Source: CAD feature listing. Evaluate the final solid. Frame: model axes, mm. Give positions to 0.01 mm unless a question says otherwise; leave off trailing zeros. Order: outer loops, then holes, each group sorted by start corner. A loop starts at its lowest first (then second) coordinate and runs counter-clockwise, first axis right, second up.
from build123d import *

# Parameters (mm, degrees)
BOSS_EXTRUDE1_DEPTH      = 5
SKETCH2_W                = 5
SKETCH2_H                = 22.5
BOSS_EXTRUDE2_DEPTH      = 38
SKETCH5_W                = 25
SKETCH5_H                = 5
BOSS_EXTRUDE3_DEPTH      = 30
FILLET3_R                = 5
SKETCH6_R                = 3
CUT_EXTRUDE4_DEPTH       = 172
SKETCH7_W                = 5
SKETCH7_H                = 22.5
BOSS_EXTRUDE4_DEPTH      = 51.5
SKETCH3_R                = 1.3
CUT_EXTRUDE2_DEPTH       = 357.71872673
SKETCH9_W                = 116
SKETCH9_H                = 63.779574991
CUT_EXTRUDE6_DEPTH       = 10
SKETCH10_W               = 25
SKETCH10_H               = 5
BOSS_EXTRUDE5_DEPTH      = 70
BOSS_EXTRUDE6_DEPTH      = 25
SKETCH12_W               = 25
SKETCH12_H               = 5
BOSS_EXTRUDE7_DEPTH      = 19.72
BOSS_EXTRUDE8_DEPTH      = 15
BOSS_EXTRUDE8_DEPTH_BACK = 4
CUT_EXTRUDE7_DEPTH       = 15
SKETCH15_R               = 2.25
CUT_EXTRUDE8_DEPTH       = 20
SKETCH16_W               = 6
SKETCH16_H               = 3
BOSS_EXTRUDE9_DEPTH      = 12.4
SKETCH17_R               = 1
CUT_EXTRUDE9_DEPTH       = 282.347152812
SKETCH27_W               = 25.232191294
SKETCH27_H               = 19
BOSS_EXTRUDE11_DEPTH     = 3
FILLET4_R                = 5
SKETCH18_R               = 2.25
CUT_EXTRUDE10_DEPTH      = 378.078044336
SKETCH19_W               = 4.5
SKETCH19_H               = 6
CUT_EXTRUDE12_DEPTH      = 383.13686347
FILLET6_R                = 10
SKETCH21_W               = 27
SKETCH21_H               = 70
CUT_EXTRUDE14_DEPTH      = 383.13686347
FILLET7_R                = 10
FILLET8_R                = 2.5
SKETCH22_R               = 2.25
CUT_EXTRUDE16_DEPTH      = 10
SKETCH23_W               = 17.043474802
SKETCH23_H               = 5.138762975
BOSS_EXTRUDE10_DEPTH     = 7
CUT_EXTRUDE17_REACH      = 372.436
CUT_EXTRUDE18_REACH      = 380.086
SKETCH25_R               = 2.25
SKETCH28_R               = 2.25
CUT_EXTRUDE19_DEPTH      = 384.936136276


with BuildPart() as part:
    # Sketch1 → Boss-Extrude1 (new body)
    with BuildSketch(Plane(origin=(0, 0, 0), x_dir=(1, 0, 0), z_dir=(0, 1, 0))):
        Polygon((0, 0), (0, -300), (186, -300), (186, 0), (176, 0), (151, 0), (151, -56.115865257), (35, -56.115865257), (35, 0), (10, 0), align=None)
    extrude(amount=BOSS_EXTRUDE1_DEPTH)

    # Sketch2 → Boss-Extrude2 (add)
    with BuildSketch(Plane.XZ):
        with Locations((53, 82.75)):
            Rectangle(SKETCH2_W, SKETCH2_H)
        with Locations((133, 82.75)):
            Rectangle(SKETCH2_W, SKETCH2_H)
    extrude(amount=BOSS_EXTRUDE2_DEPTH)

    # Sketch5 → Boss-Extrude3 (add)
    with BuildSketch(Plane.XZ):
        with Locations((173.5, 297.5)):
            Rectangle(SKETCH5_W, SKETCH5_H)
        with Locations((173.5, 242.5)):
            Rectangle(SKETCH5_W, SKETCH5_H)
        with Locations((173.5, 187.5)):
            Rectangle(SKETCH5_W, SKETCH5_H)
        with Locations((173.5, 132.5)):
            Rectangle(SKETCH5_W, SKETCH5_H)
    extrude(amount=BOSS_EXTRUDE3_DEPTH)

    # Fillet3
    fillet3_edges = [part.edges().sort_by_distance(p)[0] for p in [
        (173.5, 0, 295),
        (173.5, 0, 240),
        (173.5, 0, 185),
        (173.5, 0, 130),
    ]]
    fillet(fillet3_edges, radius=FILLET3_R)

    # Sketch6 → Cut-Extrude4 (cut)
    with BuildSketch(Plane.XY.offset(300)):
        with Locations((178, -24)):
            Circle(SKETCH6_R)
    extrude(amount=-CUT_EXTRUDE4_DEPTH, mode=Mode.SUBTRACT)

    # Sketch7 → Boss-Extrude4 (add)
    with BuildSketch(Plane.XZ):
        with Locations((2.5, 11.25)):
            Rectangle(SKETCH7_W, SKETCH7_H)
        with Locations((183.5, 11.25)):
            Rectangle(SKETCH7_W, SKETCH7_H)
    extrude(amount=BOSS_EXTRUDE4_DEPTH)

    # Sketch3 → Cut-Extrude2 (cut, through all)
    with BuildSketch(Plane(origin=(186, 0, 0), x_dir=(0, 0, -1), z_dir=(1, 0, 0))):
        with Locations((-74, -32.9)):
            Circle(SKETCH3_R)
        with Locations((-91.5, -32.9)):
            Circle(SKETCH3_R)
        with Locations((-20, -46.4)):
            Circle(SKETCH3_R)
        with Locations((-2.5, -46.4)):
            Circle(SKETCH3_R)
    extrude(amount=-CUT_EXTRUDE2_DEPTH, mode=Mode.SUBTRACT)

    # Sketch9 → Cut-Extrude6 (cut)
    with BuildSketch(Plane.XZ):
        with Locations((93, 31.889787496)):
            Rectangle(SKETCH9_W, SKETCH9_H)
    extrude(amount=-CUT_EXTRUDE6_DEPTH, mode=Mode.SUBTRACT)

    # Sketch10 → Boss-Extrude5 (add)
    with BuildSketch(Plane.XZ.offset(30)):
        with Locations((173.5, 297.5)):
            Rectangle(SKETCH10_W, SKETCH10_H)
        with Locations((173.5, 132.5)):
            Rectangle(SKETCH10_W, SKETCH10_H)
    extrude(amount=BOSS_EXTRUDE5_DEPTH)

    # Sketch11 → Boss-Extrude6 (add)
    with BuildSketch(Plane(origin=(186, 0, 0), x_dir=(0, 0, -1), z_dir=(1, 0, 0))):
        Polygon((-300, -100), (-304.901863346, -134.643852153), (-300, -135.337431613), (-295, -100), align=None)
    extrude(amount=-BOSS_EXTRUDE6_DEPTH)

    # Sketch12 → Boss-Extrude7 (add)
    with BuildSketch(Plane.XZ.offset(100)):
        with Locations((173.5, 132.5)):
            Rectangle(SKETCH12_W, SKETCH12_H)
    extrude(amount=BOSS_EXTRUDE7_DEPTH)

    # Sketch13 → Boss-Extrude8 (add, two sides: drawn at the far end of the back side and taken through both)
    with BuildSketch(Plane(origin=(0, 0, 130), x_dir=(-1, 0, 0), z_dir=(0, 0, -1)).offset(-BOSS_EXTRUDE8_DEPTH_BACK)):
        Polygon((-186, -115.314128401), (-186, -119.72), (-161, -123.135183378), (-161, -115.314128401), align=None)
    extrude(amount=BOSS_EXTRUDE8_DEPTH + BOSS_EXTRUDE8_DEPTH_BACK)

    # Sketch14 → Cut-Extrude7 (cut)
    with BuildSketch(Plane(origin=(19.462480736, -142.470246704, 0), x_dir=(0.9907978149243062, 0.13535024913615948, 0), z_dir=(0.13535024913615948, -0.9907978149243062, 0))):
        Polygon((186.357631366, 115), (168.084261749, 132.037436989), (198.015187573, 130.430954629), (197.515117956, 111.366582762), (186.357631366, 109.607523038), align=None)
    extrude(amount=-CUT_EXTRUDE7_DEPTH, mode=Mode.SUBTRACT)

    # Sketch15 → Cut-Extrude8 (cut)
    with BuildSketch(Plane(origin=(0, 39.65203451, 280.240211564), x_dir=(1, 0, 0), z_dir=(0, 0.14009757598944012, 0.9901377021414158))):
        with Locations(Location((178, -168.031966348, 0), (0, 0, 270))):
            Circle(SKETCH15_R)
        with Locations(Location((169, -149.043043011, 0), (0, 0, 270))):
            Circle(SKETCH15_R)
    extrude(amount=-CUT_EXTRUDE8_DEPTH, mode=Mode.SUBTRACT)

    # Sketch16 → Boss-Extrude9 (add)
    with BuildSketch(Plane.XZ):
        with Locations((169, 273.5)):
            Rectangle(SKETCH16_W, SKETCH16_H)
        with Locations((140.4, 273.5)):
            Rectangle(SKETCH16_W, SKETCH16_H)
        with Locations((169, 218.5)):
            Rectangle(SKETCH16_W, SKETCH16_H)
        with Locations((169, 163.5)):
            Rectangle(SKETCH16_W, SKETCH16_H)
        with Locations((140.4, 218.5)):
            Rectangle(SKETCH16_W, SKETCH16_H)
        with Locations((140.4, 163.5)):
            Rectangle(SKETCH16_W, SKETCH16_H)
    extrude(amount=BOSS_EXTRUDE9_DEPTH)

    # Sketch17 → Cut-Extrude9 (cut, through all)
    with BuildSketch(Plane(origin=(0, 0, 162), x_dir=(-1, 0, 0), z_dir=(0, 0, -1))):
        with BuildLine():
            ThreePointArc((-169.75, -5.6), (-169.95, -6.2), (-169.75, -6.8))
            ThreePointArc((-169.75, -6.8), (-168.633772234, -7.148683298), (-167.95, -6.2))
            ThreePointArc((-167.95, -6.2), (-168.633772234, -5.251316702), (-169.75, -5.6))
        make_face()
        with Locations((-140.45, -6.2)):
            Circle(SKETCH17_R)
    extrude(amount=-CUT_EXTRUDE9_DEPTH, mode=Mode.SUBTRACT)

    # Sketch27 → Boss-Extrude11 (add)
    with BuildSketch(Plane(origin=(19.462480736, -142.470246704, 0), x_dir=(0.9907978149243062, 0.13535024913615953, 0), z_dir=(0.13535024913615953, -0.9907978149243062, 0))):
        with Locations((155.468166102, 124.5)):
            Rectangle(SKETCH27_W, SKETCH27_H)
    extrude(amount=BOSS_EXTRUDE11_DEPTH)

    # Fillet4
    fillet4_edges = [part.edges().sort_by_distance(p)[0] for p in [
        (140.4, 0, 220),
        (169, 0, 165),
        (169, 0, 220),
        (140.4, 0, 275),
        (140.4, 0, 165),
        (169, 0, 275),
    ]]
    fillet(fillet4_edges, radius=FILLET4_R)

    # Sketch18 → Cut-Extrude10 (cut, through all)
    with BuildSketch(Plane(origin=(0, -115.314128401, 0), x_dir=(1, 0, 0), z_dir=(0, 1, 0))):
        with Locations(Location((174.885718372, -120.99470656, 0), (0, 0, 180))):
            Circle(SKETCH18_R)
    extrude(amount=-CUT_EXTRUDE10_DEPTH, mode=Mode.SUBTRACT)

    # Sketch19 → Cut-Extrude12 (cut, through all)
    with BuildSketch(Plane.XZ):
        with Locations((144.95, 82.75)):
            Rectangle(SKETCH19_W, SKETCH19_H)
        with Locations((41.05, 82.75)):
            Rectangle(SKETCH19_W, SKETCH19_H)
    extrude(amount=-CUT_EXTRUDE12_DEPTH, mode=Mode.SUBTRACT)

    # Fillet6
    fillet6_edges = [part.edges().sort_by_distance(p)[0] for p in [
        (35, 2.5, 63.779574991),
        (151, 2.5, 63.779574991),
    ]]
    fillet(fillet6_edges, radius=FILLET6_R)

    # Sketch21 → Cut-Extrude14 (cut, through all)
    with BuildSketch(Plane.XZ):
        with Locations((13.5, 83)):
            Rectangle(SKETCH21_W, SKETCH21_H)
        with Locations((172.5, 83)):
            Rectangle(SKETCH21_W, SKETCH21_H)
    extrude(amount=-CUT_EXTRUDE14_DEPTH, mode=Mode.SUBTRACT)

    # Fillet7
    fillet7_edges = [part.edges().sort_by_distance(p)[0] for p in [
        (27, 2.5, 118),
        (27, 2.5, 48),
        (159, 2.5, 48),
        (159, 2.5, 118),
    ]]
    fillet(fillet7_edges, radius=FILLET7_R)

    # Fillet8
    fillet8_edges = [part.edges().sort_by_distance(p)[0] for p in [
        (55.5, 0, 82.75),
        (130.5, 0, 82.75),
    ]]
    fillet(fillet8_edges, radius=FILLET8_R)

    # Sketch22 → Cut-Extrude16 (cut)
    with BuildSketch(Plane.XZ):
        with Locations(Location((123, 76.044790491, 0), (0, 0, 270))):
            Circle(SKETCH22_R)
        with Locations(Location((63, 76.044790491, 0), (0, 0, 270))):
            Circle(SKETCH22_R)
        with Locations(Location((24.5, 25.25, 0), (0, 0, 270))):
            Circle(SKETCH22_R)
        with Locations(Location((161.5, 25.617459027, 0), (0, 0, 270))):
            Circle(SKETCH22_R)
    extrude(amount=-CUT_EXTRUDE16_DEPTH, mode=Mode.SUBTRACT)

    # Sketch23 → Boss-Extrude10 (add)
    with BuildSketch(Plane.XY.offset(135)):
        with Locations((169.584553608, -121.006176699)):
            Rectangle(SKETCH23_W, SKETCH23_H)
    extrude(amount=BOSS_EXTRUDE10_DEPTH)

    # Sketch24 → Cut-Extrude17 (cut, up to next)
    with BuildSketch(Plane.ZY.offset(-161.062816207), mode=Mode.PRIVATE) as cut_extrude17_sk1:
        Polygon((142, -121.648432415), (135, -122.638883571), (134.714975443, -124.33810847), (142, -124.33810847), align=None)
    cut_extrude17_tool1 = extrude(cut_extrude17_sk1.sketch, amount=-CUT_EXTRUDE17_REACH, mode=Mode.PRIVATE) & part.part
    add(cut_extrude17_tool1.solids().sort_by_distance((161.062816, -123.230784, 138.703404))[0], mode=Mode.SUBTRACT)

    # Cut-Extrude18: up to this plane
    cut_extrude18_end = Plane(origin=(186.407050747, -121.648432415, 142), z_dir=(0, 0.9901377021414159, -0.14009757598943937))
    # Sketch25 → Cut-Extrude18 (cut, up to the surface)
    with BuildSketch(Plane(origin=(0, -118.436795211, 0), x_dir=(1, 0, 0), z_dir=(0, 1, 0)), mode=Mode.PRIVATE) as cut_extrude18_sk1:
        with Locations(Location((174.719138996, -138.089405518, 0), (0, 0, 270))):
            Circle(SKETCH25_R)
    cut_extrude18_tool1 = split(extrude(cut_extrude18_sk1.sketch, amount=-CUT_EXTRUDE18_REACH, mode=Mode.PRIVATE), bisect_by=cut_extrude18_end, keep=Keep.BOTH, mode=Mode.PRIVATE)
    add(cut_extrude18_tool1.solids().sort_by_distance((174.719139, -118.436795, 138.089406))[0], mode=Mode.SUBTRACT)

    # Sketch28 → Cut-Extrude19 (cut, through all)
    with BuildSketch(Plane(origin=(0, 5, 0), x_dir=(1, 0, 0), z_dir=(0, 1, 0))):
        with Locations(Location((93, -260, 0), (0, 0, 270))):
            Circle(SKETCH28_R)
    extrude(amount=-CUT_EXTRUDE19_DEPTH, mode=Mode.SUBTRACT)


solid = part.part
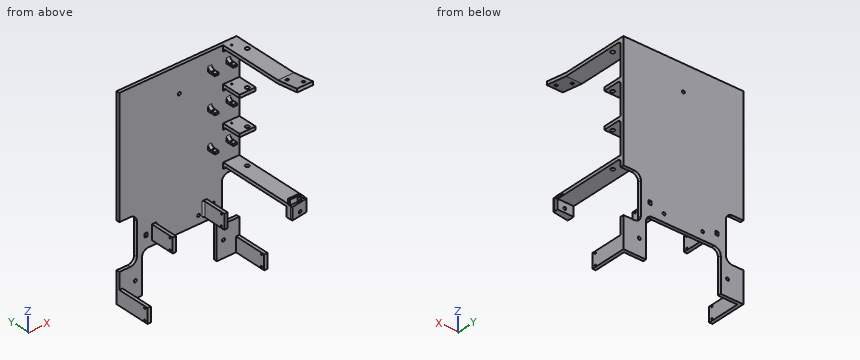
1) Section query B-B on x = 74.5. Output: boundary loops of the cut face in (y, z), and give its area (3 significant figures).
Checks:
outline: (0, 63.78) - (5, 63.78) - (5, 300) - (0, 300) - close
area: 1,180 mm2
2) Section query A-A on y = -41.5. Output: boundary loops of the cut face in (x, z), and give its area (3 significant figures).
Checks:
outline: (0, 0) - (5, 0) - (5, 22.5) - (0, 22.5) - close; (161, 130) - (186, 130) - (186, 135) - (161, 135) - close; (161, 295) - (186, 295) - (186, 300) - (161, 300) - close; (181, 0) - (186, 0) - (186, 22.5) - (181, 22.5) - close
area: 475 mm2
3) Section query C-C on z = 207. Output: boundary loops of the cut face in (x, y), and give its area (3 significant figures).
Checks:
outline: (0, 0) - (186, 0) - (186, 5) - (0, 5) - close
area: 930 mm2
4) Ray query, L1, parallel to Z at x = 173.5, y = -28.5; L2, parallel to Y at x = 184, z = 20; L3, parallel to Z at x = 51, y = -32. Return the intervals inside material, ascending.
Checks:
L1: z = 130 to 135, 185 to 190, 240 to 245, 295 to 300
L2: y = -51.5 to -47.7, -45.1 to 5
L3: z = 71.5 to 73.06, 74.94 to 90.56, 92.44 to 94
5) First-contact query: pin 1 Ø2.5 at (x, z) = (93, 260) entering from +Y; pin 2 Ø4 at (y, z) = (-7, 166) entering from -X; pin 3 Ø1.5 at (y, z) = (1.5, 82.5) entering from -X; pin 4 Ø8 at (x, y) = (178, -24) entering from +Z. Flat tips, straight axial feed; report the tip coordinate or a pass-through.
Checks:
pin 1: passes through
pin 2: stops at x = 137.4
pin 3: stops at x = 27
pin 4: stops at z = 300
